Drawing for the job (mm, zero at the part's lowest x, y, z). Round coordinates to 2 decimals unless told otherwise and drop trailing zeros. Order: outer loops, then holes, each group sorted by start corner. A loop starts at its lowest first (then second) coordinate and runs counter-clockwise, first axis right, second up. Notation, with made-up numbers: M -11.5,67 L 38.5,67 A34 cw 38.5,103 Z; hole C -24,-14.75 d10. An arc over 180 degrees is marked long. One line per item, written item: value. Start each with the question number.
Item 1: Band-saw the part on B-B, the plane x = 147.5. Write the cut outline in (y, z), then the cut area to 3 significant figures.
Item 2: Pin check, flat tips, straight feed: pin 1 (0.9 mm diameter, centred on x = 97, y = 0.5, fed in from +Z); pin 2 (1 mm diameter, centred on y = 12, z = 1.5, fed in from +X); pin 3 (1.5 mm diameter, centred on y = 11, z = 11.5, fed in from -X). Stop position of each tip, or through.
Item 3: Probe L1, parallel to X at y = 11.75, z = 6; L2, parallel to Y at x = 76.5, z = 6.25 (1 decimal); L3, parallel to Y at x = 127.5, z = 8.75 (1 decimal). List the from-to ranges inside material, lowest first.
Item 4: Band-saw the part on A-A, the plane z = 6.35. Write the cut outline in (x, y), then the cut area to 3 significant figures.
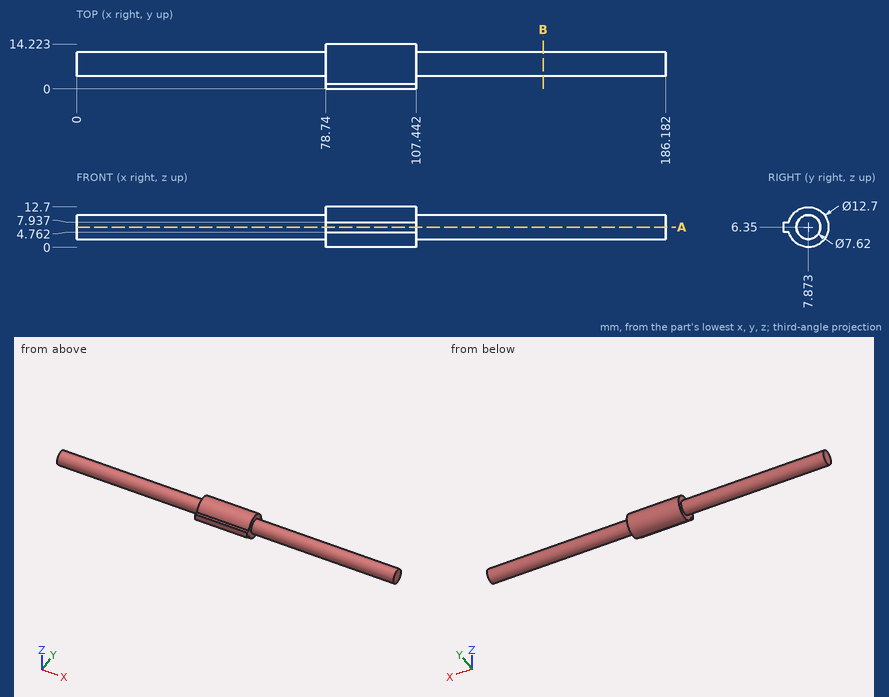
Output:
1. outline: C 7.87,6.35 d7.62
1. area: 45.6 mm²
2. pin 1: stops at z = 7.94
2. pin 2: stops at x = 107.44
2. pin 3: stops at x = 78.74
3. L1: x = 78.74 to 107.44
3. L2: y = 4.1 to 11.7
3. L3: y = 4.9 to 10.8
4. outline: M 0,4.06 L 78.74,4.06 L 78.74,0 L 107.44,0 L 107.44,4.06 L 186.18,4.06 L 186.18,11.68 L 107.44,11.68 L 107.44,14.22 L 78.74,14.22 L 78.74,11.68 L 0,11.68 Z
4. area: 1,610 mm²
